For this review, take the finished solid that the model builds, in its own axes (mm). A direction names the side the tool comes from. Round coordinates to 2 decimals unless told otherwise and drop trailing zeros. Write each loop counter-clockwise with the first axis right and the second up, starting at its lowest first coordinate (ties: lowest second). Pieces come first, ordered by that corner, then holes.
from build123d import *


with BuildPart() as f1:
    # F0 (on Front) → F1 (revolve)
    with BuildSketch(Plane.XZ):
        with BuildLine():
            Line((13, -25), (15.1172224432, -25))
            Line((15.1172224432, -25), (15.1172224432, -2.5685927831))
            Line((15.1172224432, -2.5685927831), (15.1172224432, 2.5685927831))
            Line((15.1172224432, 2.5685927831), (15.1172224432, 35))
            add(Edge.make_bspline(
                [(15.1172224432, 35), (10.0791664263, 34.3889759882), (4.0376053781, 22.9443653974), (8.016607968, 17.2045025786), (9.5755117753, 12.7803640445)],
                knots=[0, 0, 0, 0, 0.5233807249, 1, 1, 1, 1], degree=3))
            Line((9.5755117753, 12.7803640445), (13, 0))
            Line((13, 0), (13, -25))
        make_face()
        Polygon((15.1172224432, 2.5685927831), (15.1172224432, -2.5685927831), (19.6100920439, -2.5685927831), (19.6100920439, 0), (19.6100920439, 2.5685927831), align=None)
    revolve(axis=Axis((0, 0, -12.5), (0, 0, -1)))


solid = f1.part
(1) We need section A-A, the plane z = -13.5. Give the boundary of the cut face in (x, y), and give its area (3 significant figures).
Geometry check:
outline: circle Ø30.23 at (0, 0); hole circle Ø26 at (0, 0)
area: 187 mm2
(2) We need section B-B, the plane x = 17. Give the boundary of the cut face in (y, z).
Geometry check:
outline: (-9.78, -2.57) - (9.78, -2.57) - (9.78, 2.57) - (-9.78, 2.57) - close
(3) For pin 1 Ø10 at (x, z) = (6, 7) entering from +Y; pin 2 Ø3 at (x, z) = (-5, -11) entering from -Y; pin 3 Ø3 at (x, z) = (4, 9) entering from -Y, all flat-tipped, find the tip position at first contact; note any pin that passes through.
Geometry check:
pin 1: stops at y = 19.26
pin 2: stops at y = -14.71
pin 3: stops at y = -14.91
(4) For line 1 along Y through (x, z) = (0, -10); line 2 along Z through (x, y) = (-16, 2), list the stretches that pass through material, from the lowest coordinate up.
Geometry check:
line 1: y = -15.12 to -13, 13 to 15.12
line 2: z = -2.57 to 2.57
(5) For faces 4 (the face through (-4.251, 19.144, 0.036)), 5 (the face through (-10, 12, -2.569)), list the 3-axis set-ups (+Z, -Z, +X, -X, +Y, -Y) from which the entire face can be reached by the end or side of a thin tool; tool diameter is ignored.
Geometry check:
face 4: +Z, -Z
face 5: -Z
(6) Mouldability with a two-part tool opening along X and no side actions: class faces 1 (the face through (10, 12, 2.569)), 2 (the face through (-15.1, -0.7, 19)), 3 (the face through (-10.316, 7.91, -12.675)) as pulls with the +X half, pulls with the -X half, needs draft (parallel to the pull), parting line crosses it, or undercut.
Geometry check:
face 1: needs draft
face 2: parting line crosses it
face 3: undercut
